Design review of the part built by this model. Coordinates are the model's own, in mm. Face numbers are marked on the shaded views. A direction names the side the tool comes from. Coordinates: 2 decimals unless noted, no trailing zeros. Write each loop counter-clockwise with the first axis right and the second up, starting at its lowest first coordinate (ties: lowest second). Pieces come first, ordered by that corner, then holes.
Q1. Take a section at B-B, the plane z = 26. Write out the cut boundary in (x, y).
Q2. Take a section at C-C, the plane y = -21.5. Write out the cut boundary in (x, z).
Q3. For L1, parallel to X at y = 46, z = -6; L2, parallel to Y at x = 0, z = -39; L3, parallel to Z at x = -10, y = 33, list the stretches that pass through material, from the lowest coordinate up.
Q4. The part is to be moulded in two halves that separate along X. For the marked faces 1, 2, 3 and 4, say which applies: released by +X, released by -X, zero draft, split by the parting line, or undercut.
Q5. For pin 1 Ø6 at (x, z) = (14.5, 31.5) entering from -Y, flat-tipped, find the tip position at first contact; note if it passes through.
Q6. Take a section at A-A, the plane x = 0. Write out the cut boundary in (y, z).
Q7. Take a section at D-D, the plane y = 27.5. Write out the cut boundary in (x, z), plus the area to 3 significant figures.
Q8. For the marked faces 5 and 6, list the 3-axis set-ups (+Z, -Z, +X, -X, +Y, -Y) from which the entire face can be reached by the end or side of a thin tool; tool diameter is ignored.
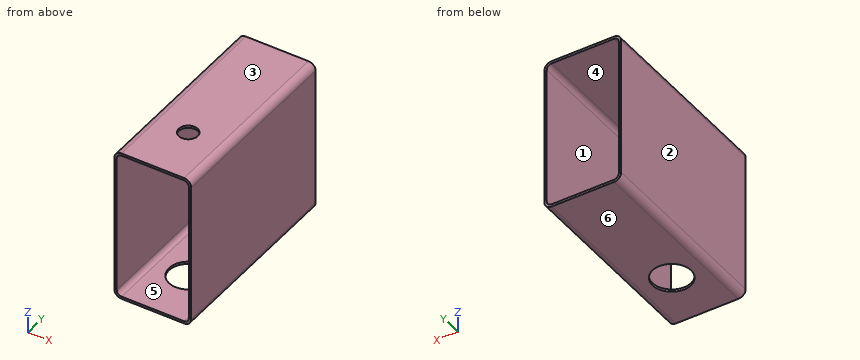
Autodesk Inventor part; units mm, degrees
ref_plane "YZ Plane" through (0, 0, 0) normal (1, 0, 0) x (0, 1, 0)
ref_plane "XZ Plane" through (0, 0, 0) normal (0, 1, 0) x (-1, 0, 0)
ref_plane "XY Plane" through (0, 0, 0) normal (0, 0, 1) x (1, 0, 0)
sketch "Sketch1" plane through (0, 0, 0) normal (0, 1, 0) x (-1, 0, 0)
  line L0 (-20, 40) -> (20, 40)
  line L1 (20, 40) -> (20, -40)
  line L2 (20, -40) -> (-20, -40)
  line L3 (-20, -40) -> (-20, 40)
  line L4 (-20, 40) -> (20, -40) construction
  line L5 (20, 40) -> (-20, -40) construction
  line L6 (-17.5, 37.5) -> (17.5, -37.5) construction
  line L7 (18.764, 38.7789) -> (-17.2638, -35.6785) construction
  line L8 (18.75, 38.75) -> (-18.75, 38.75)
  line L9 (-18.75, 38.75) -> (-18.75, -38.75)
  line L10 (-18.75, -38.75) -> (18.75, -38.75)
  line L11 (18.75, -38.75) -> (18.75, 38.75)
  line L12 (18.75, 38.75) -> (-18.75, -38.75) construction
  line L13 (-18.75, 38.75) -> (18.75, -38.75) construction
  point P0 (0, 0)
  dimension "d0" = 40
  dimension "d1" = 80
  dimension "d33" = 37.5
  dimension "d34" = 77.5
extrude "Extrusion1" add sketch "Sketch1" along normal mid plane 100
fillet "Fillet1" radius 3.75 4 edges at (20, 0, -40) (20, 0, 40) (-20, 0, -40) (-20, 0, 40)
fillet "Fillet1" radius 2.5 4 edges at (-18.75, 0, -38.75) (18.75, 0, 38.75) (18.75, 0, -38.75) (-18.75, 0, 38.75)
sketch "Sketch2" plane through (16.25, 50, -40) normal (0, 0, -1) x (-1, 0, 0)
  line L0 (32.5, -100) -> (0, -100)
  line L1 (16.25, -100) -> (16.25, -71.5)
  circle A0 centre (16.25, -71.5) radius 4.95
  circle A1 centre (16.25, -71.5) radius 10
  point P0 (16.25, -50)
  dimension "d10" = 28.5
  dimension "d11" = 9.9
  dimension "d12" = 20
extrude "Extrusion2" cut sketch "Sketch2" against normal through all contours A0
sketch "Sketch3" plane through (16.25, 50, -40) normal (0, 0, -1) x (-1, 0, 0)
  circle A0 centre (16.25, -71.5) radius 4.95
  circle A1 centre (16.25, -71.5) radius 10
  point P0 (16.25, -50)
  dimension "d15" = 20
extrude "Extrusion3" cut sketch "Sketch3" against normal blind 10
properties part number "tubo1-40x40x640" material "Aluminum"
Responses:
1. outline: (-20, -50) - (-18.75, -50) - (-18.75, 50) - (-20, 50) - close; (18.75, -50) - (20, -50) - (20, 50) - (18.75, 50) - close
2. outline: (-20, -36.25) arc R3.75 ccw to (-16.25, -40) - (-10, -40) - (-10, -38.75) - (-16.25, -38.75) arc R2.5 cw to (-18.75, -36.25) - (-18.75, 36.25) arc R2.5 cw to (-16.25, 38.75) - (-4.95, 38.75) - (-4.95, 40) - (-16.25, 40) arc R3.75 ccw to (-20, 36.25) - close; (4.95, 38.75) - (16.25, 38.75) arc R2.5 cw to (18.75, 36.25) - (18.75, -36.25) arc R2.5 cw to (16.25, -38.75) - (10, -38.75) - (10, -40) - (16.25, -40) arc R3.75 ccw to (20, -36.25) - (20, 36.25) arc R3.75 ccw to (16.25, 40) - (4.95, 40) - close
3. L1: x = -20 to -18.75, 18.75 to 20
3. L2: y = -50 to -31.5, -11.5 to 50
3. L3: z = -40 to -38.75, 38.75 to 40
4. face 1: undercut
4. face 2: released by -X
4. face 3: zero draft
4. face 4: undercut
5. pin 1: passes through
6. outline: (-50, -40) - (-31.5, -40) - (-31.5, -38.75) - (-50, -38.75) - close; (-50, 38.75) - (-26.45, 38.75) - (-26.45, 40) - (-50, 40) - close; (-16.55, 38.75) - (50, 38.75) - (50, 40) - (-16.55, 40) - close; (-11.5, -40) - (50, -40) - (50, -38.75) - (-11.5, -38.75) - close
7. outline: (-20, -36.25) arc R3.75 ccw to (-16.25, -40) - (16.25, -40) arc R3.75 ccw to (20, -36.25) - (20, 36.25) arc R3.75 ccw to (16.25, 40) - (-16.25, 40) arc R3.75 ccw to (-20, 36.25) - close; hole (-18.75, -36.25) arc R2.5 ccw to (-16.25, -38.75) - (16.25, -38.75) arc R2.5 ccw to (18.75, -36.25) - (18.75, 36.25) arc R2.5 ccw to (16.25, 38.75) - (-16.25, 38.75) arc R2.5 ccw to (-18.75, 36.25) - close
7. area: 287 mm2
8. face 5: +Y, -Y
8. face 6: -Z, +X, -X, +Y, -Y
